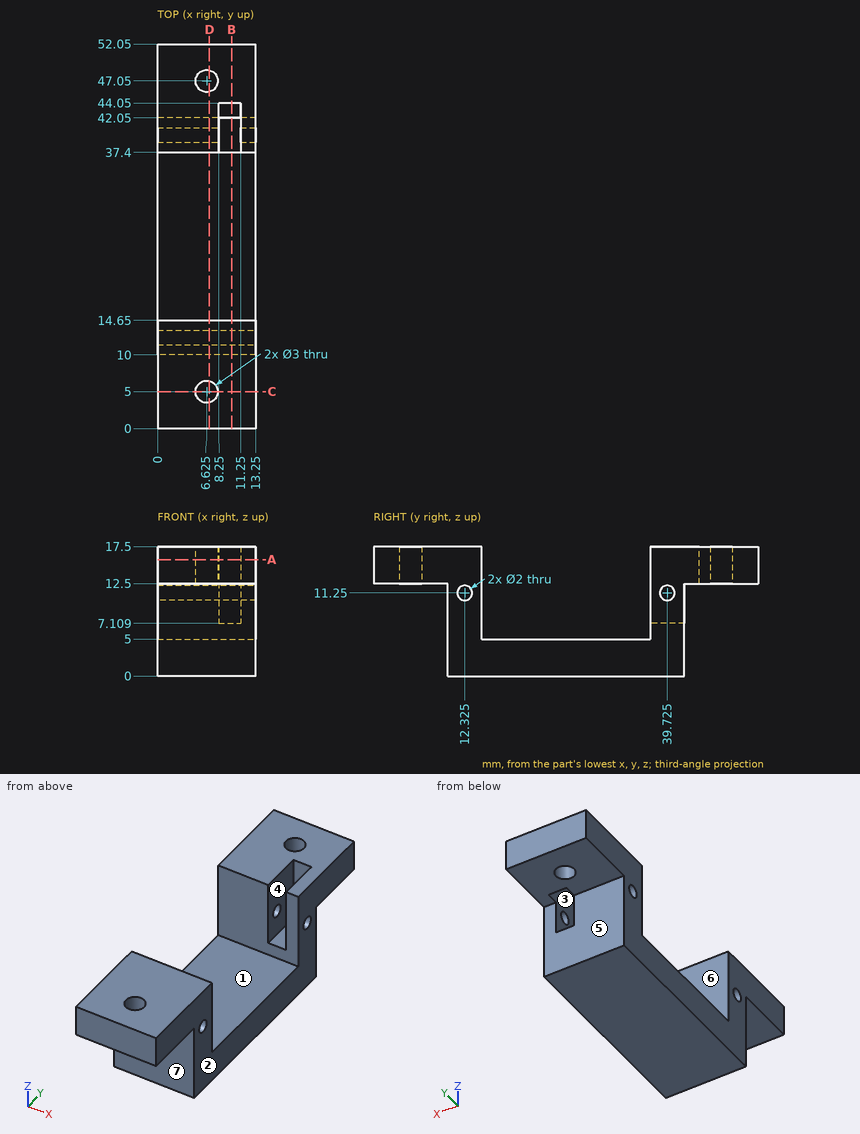
Could you check a few things on this drawing? It's one solid part, dimensions in mm from its lowest x, y, z. A direction names the side the tool comes from. Round coordinates to 2 decimals unless told otherwise and drop trailing zeros. Order: outer loops, then holes, each group sorted by start corner. A loop starts at its lowest first (then second) coordinate and runs counter-clockwise, first axis right, second up. Notation, with made-up numbers: M -33.75,-28 L -19.75,-28 A33 ccw -19.75,4 Z; hole C 44,-34.75 d3. An arc over 180 degrees is marked long. One line per question, with ' | ' between items. Start each with the question number.
(1) Suppose I cut it at A-A on z = 15.75. List the corners of the cut face in (x, y) for me (3 decimals), then the cut area to 3 significant figures.
(2) Please list where these lines run through material, in increasing order: line 1 along Y through (x, z) = (12.8, 11.25) (3 decimals); line 2 along X through (y, z) = (39, 12); line 3 along Y through (x, z) = (4.5, 14.5).
(3) For P1, Ø1.5, axis at x = 2.5, z = 7, coming from the -Y side; P2, Ø1.8, axis at y = 39.725, z = 11.25, coming from the -X side; P3, Ø4, axis at x = 5.5, y = 45.5, coming from the -Z side, each with a flat end and sliding along its axis, tell me the tip position at first contact or that it passes through.
(4) Suppose I cut it at C-C on y = 5. List the corners of the cut face in (x, z) for me (3 decimals), then the cut area to 4 significant figures.
(5) For the marked faces 5, 6 and 7, which set-ups out of +Z, -Z, +X, -X, +Y, -Y let a thin tool reach every point of the face, with its end or its side?
(6) Thinking about a two-plate mould opening in X: for the marked faces 1, 2, 3 and 4, which applies, +X half, -X half, draft (parallel to the pull), parting line (faces both ways), or undercut?
(7) Suppose I cut it at B-B on x = 10. List the corners of the cut face in (y, z) for me (3 decimals).
(8) Suppose I cut it at D-D on x = 7. List the corners of the cut face in (y, z) for me (3 decimals).
Geometry results:
1) outline: M 0,0 L 13.25,0 L 13.25,14.65 L 0,14.65 Z; M 0,37.4 L 8.25,37.4 L 8.25,44.05 L 11.25,44.05 L 11.25,37.4 L 13.25,37.4 L 13.25,52.05 L 0,52.05 Z; hole C 6.625,5 d3; hole C 6.625,47.05 d3 | area: 354 mm²
2) line 1: 10 to 11.325, 13.325 to 14.65, 37.4 to 38.725, 40.725 to 42.05 | line 2: 0 to 8.25, 11.25 to 13.25 | line 3: 0 to 14.65, 37.4 to 52.05
3) P1: y = 10 | P2: through | P3: z = 12.5
4) outline: M 0,12.5 L 5.125,12.5 L 5.125,17.5 L 0,17.5 Z; M 8.125,12.5 L 13.25,12.5 L 13.25,17.5 L 8.125,17.5 Z | area: 51.25 mm²
5) face 5: -Z, +X, -X, +Y | face 6: +Z, +X, -X | face 7: -Z, +X, -X, -Y
6) face 1: draft | face 2: +X half | face 3: undercut | face 4: undercut
7) outline: M 0,12.5 L 10,12.5 L 10,0 L 42.05,0 L 42.05,7.109 L 37.4,7.109 L 37.4,5 L 14.65,5 L 14.65,17.5 L 0,17.5 Z; M 44.05,12.5 L 52.05,12.5 L 52.05,17.5 L 44.05,17.5 Z; hole C 12.325,11.25 d2
8) outline: M 0,12.5 L 3.548,12.5 L 3.548,17.5 L 0,17.5 Z; M 6.452,12.5 L 10,12.5 L 10,0 L 42.05,0 L 42.05,12.5 L 45.598,12.5 L 45.598,17.5 L 37.4,17.5 L 37.4,5 L 14.65,5 L 14.65,17.5 L 6.452,17.5 Z; M 48.502,12.5 L 52.05,12.5 L 52.05,17.5 L 48.502,17.5 Z; hole C 12.325,11.25 d2; hole C 39.725,11.25 d2
